For this review, take the finished solid that the model builds, in its own axes (mm). Face numbers are marked on the shaded views. A direction names the side the tool comes from. Give positions to 0.01 mm unless a question says otherwise; leave off trailing zeros. Loops run counter-clockwise (first coordinate to the right, second up) from the corner with the lowest first, then second, coordinate; pieces in that order, holes last. Notation, with made-up numbers: (40, 13.5) - (84, 13.5) arc R17 cw to (84, 25.5) - close; hole circle Ø8 at (44.25, 41). An arc over 180 degrees is marked (long way). Put each result on its own line as item: value.
from build123d import *

# Parameters (mm, degrees)
F0_W     = 20
F0_H     = 36
F1_DEPTH = 10
F2_R     = 3
F3_DEPTH = 3
F4_R     = 3
F5_DEPTH = 3


with BuildPart() as f1:
    # F0 (on Front) → F1 (new body)
    with BuildSketch(Plane.XZ):
        with Locations((10, 18)):
            Rectangle(F0_W, F0_H)
    extrude(amount=F1_DEPTH)

    # F2 (on face) → F3 (cut)
    with BuildSketch(Plane(origin=(0, 0, 0), x_dir=(1, 0, 0), z_dir=(0, 0, -1))):
        with Locations((10, 5)):
            Circle(F2_R)
    extrude(amount=-F3_DEPTH, mode=Mode.SUBTRACT)

    # F4 (on face) → F5 (cut)
    with BuildSketch(Plane.XY.offset(36)):
        with Locations((10, -5)):
            Circle(F4_R)
    extrude(amount=-F5_DEPTH, mode=Mode.SUBTRACT)


solid = f1.part
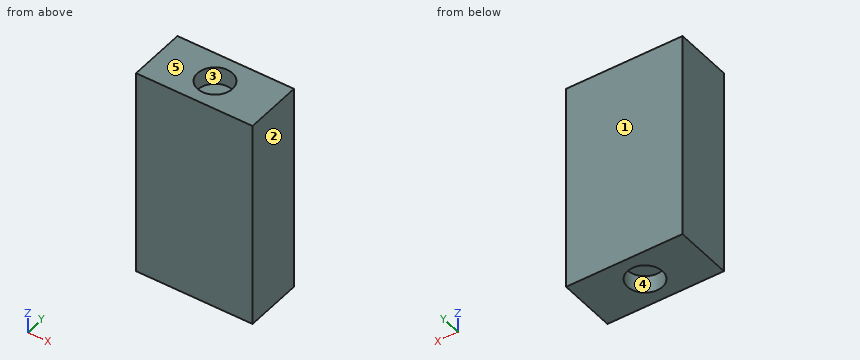
1) Insertion check: pin 1 Ø1.8 at (x, y) = (10.5, -4) entering from +Z. The pin has a flat end and moves straight along its axis. Give the tip position at first contact, or say it passes through.
Geometry check:
pin 1: stops at z = 33
2) Take a section at A-A on x = 10. State the section outline as (y, z) points.
Geometry check:
outline: (-10, 0) - (-8, 0) - (-8, 3) - (-2, 3) - (-2, 0) - (0, 0) - (0, 36) - (-2, 36) - (-2, 33) - (-8, 33) - (-8, 36) - (-10, 36) - close
3) Take a section at B-B on y = -5. State the section outline as (x, z) points, and give its area (3 significant figures).
Geometry check:
outline: (0, 0) - (7, 0) - (7, 3) - (13, 3) - (13, 0) - (20, 0) - (20, 36) - (13, 36) - (13, 33) - (7, 33) - (7, 36) - (0, 36) - close
area: 684 mm²
4) For the marked faces 4 and 5, list the 3-axis set-ups (+Z, -Z, +X, -X, +Y, -Y) from which the entire face can be reached by the end or side of a thin tool; tool diameter is ignored.
Geometry check:
face 4: -Z
face 5: +Z, +X, -X, +Y, -Y
5) Wall thickness on line 1 (X direction, y = -5, z = 2.4); line 2 (Y direction, x = 10, z = 34.55); line 3 (Z direction, x = 8.25, y = -5): over which ranges is each line inside the solid? List them lowest first.
Geometry check:
line 1: x = 0 to 7, 13 to 20
line 2: y = -10 to -8, -2 to 0
line 3: z = 3 to 33
6) Draft analysis for pull direction X (two halves, no side actions). For the marked faces 1, 2 and 3, state which applies: pulls with the +X half, pulls with the -X half, needs draft (parallel to the pull), parting line crosses it, or undercut.
Geometry check:
face 1: needs draft
face 2: pulls with the +X half
face 3: undercut
